from build123d import *

# Parameters (mm, degrees)
SKETCH2_W           = 40
SKETCH2_H           = 200
BOSS_EXTRUDE1_DEPTH = 3.175
CUT_EXTRUDE1_DEPTH  = 10
FILLET1_R           = 20
FILLET2_R           = 18
SKETCH6_R           = 2
CUT_EXTRUDE4_DEPTH  = 103.029802631
SKETCH7_R           = 2
CUT_EXTRUDE5_DEPTH  = 103.029802631


with BuildPart() as part:
    # Sketch2 → Boss-Extrude1 (new body)
    with BuildSketch(Plane.XY):
        Rectangle(SKETCH2_W, SKETCH2_H)
    extrude(amount=BOSS_EXTRUDE1_DEPTH)

    # Sketch3 → Cut-Extrude1 (cut)
    with BuildSketch(Plane(origin=(0, 0, 0), x_dir=(-1, 0, 0), z_dir=(0, 0, -1))):
        with BuildLine():
            Line((1.325, -88.501876173), (-1.325, -88.501876173))
            ThreePointArc((-1.325, -88.501876173), (0, -92), (1.325, -88.501876173))
        make_face()
    extrude(amount=-CUT_EXTRUDE1_DEPTH, mode=Mode.SUBTRACT)

    # Fillet1
    fillet1_edges = [part.edges().sort_by_distance(p)[0] for p in [
        (20, -100, 1.5875),
        (-20, -100, 1.5875),
    ]]
    fillet(fillet1_edges, radius=FILLET1_R - 0.0001)  # a hair under: the kernel refuses the full size

    # Fillet2
    fillet2_edges = [part.edges().sort_by_distance(p)[0] for p in [
        (-20, 100, 1.5875),
        (20, 100, 1.5875),
    ]]
    fillet(fillet2_edges, radius=FILLET2_R)

    # Sketch6 → Cut-Extrude4 (cut, through all)
    with BuildSketch(Plane.XY.offset(3.175)):
        with Locations((15, 67)):
            Circle(SKETCH6_R)
        with Locations((15, -21)):
            Circle(SKETCH6_R)
        with Locations((15, 23)):
            Circle(SKETCH6_R)
        with Locations((15, -65)):
            Circle(SKETCH6_R)
        with Locations(Location((-15, -65, 0), (0, 0, 180))):
            Circle(SKETCH6_R)
        with Locations(Location((-15, 23, 0), (0, 0, 180))):
            Circle(SKETCH6_R)
        with Locations(Location((-15, -21, 0), (0, 0, 180))):
            Circle(SKETCH6_R)
        with Locations(Location((-15, 67, 0), (0, 0, 180))):
            Circle(SKETCH6_R)
    extrude(amount=-CUT_EXTRUDE4_DEPTH, mode=Mode.SUBTRACT)

    # Sketch7 → Cut-Extrude5 (cut, through all)
    with BuildSketch(Plane.XY.offset(3.175)):
        with Locations((-12, 88)):
            Circle(SKETCH7_R)
        with Locations((12, 88)):
            Circle(SKETCH7_R)
    extrude(amount=-CUT_EXTRUDE5_DEPTH, mode=Mode.SUBTRACT)


solid = part.part
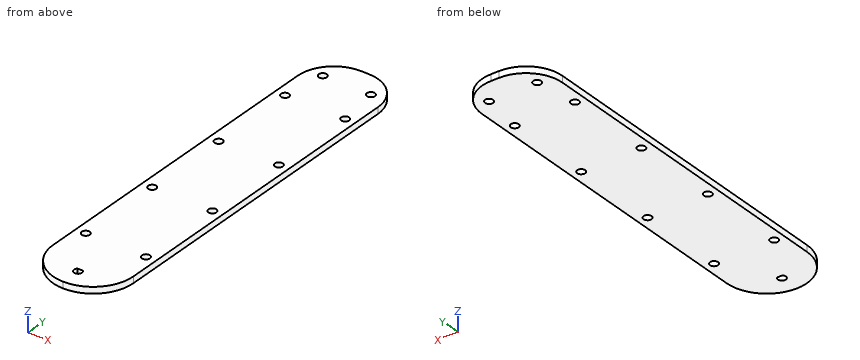
Part model, mm, in its own coordinate system. Coordinates: 2 decimals unless noted, no trailing zeros. Loops run counter-clockwise (first coordinate to the right, second up) from the corner with the lowest first, then second, coordinate; pieces in that order, holes last. Notation, with made-up numbers: M 33,88 L 55,88 A20 cw 55,127 Z; hole C 81,-31 d6. An arc over 180 degrees is marked long. Use a Markdown table: item, result. Add a question column.
Q1. Cut at B-B (z = 2.5). Give the number of separate pieces and of enclosed holes in the cut face, and give its area (3 significant figures).
Q2. Pin check, flat tips, straight feed: P1, Ø2.5, axis at x = -15, y = 67, coming from the -Z side; P2, Ø1, axis at x = 14.5, z = 3, coming from the +Y side. Stop position of each tip, or through.
Q3. Cut at A-A (y = 67). Write the cut outline in (x, z) (3 decimals), and give its area (3 significant figures).
Q4. Probe L1, parallel to Y at x = 15, z = 1.85; L2, parallel to Y at x = -12.5, z = 1.5; L3, parallel to Y at x = -4.5, z = 2.2. List the from-to ranges inside material, lowest first.
Worked out:
| question | item | result |
|---|---|---|
| 1 | separate pieces | 1 |
| 1 | enclosed holes | 11 |
| 1 | area | 7,550 mm2 |
| 2 | P1 | passes through |
| 2 | P2 | stops at y = 95.42 |
| 3 | outline | M -20,0 L -17,0 L -17,3.175 L -20,3.175 Z; M -13,0 L 13,0 L 13,3.175 L -13,3.175 Z; M 17,0 L 20,0 L 20,3.175 L 17,3.175 Z |
| 3 | area | 102 mm2 |
| 4 | L1 | y = -93.23 to -67, -63 to -23, -19 to 21, 25 to 65, 69 to 94.45 |
| 4 | L2 | y = -95.61 to 86.06, 89.94 to 96.62 |
| 4 | L3 | y = -99.49 to 99.83 |
